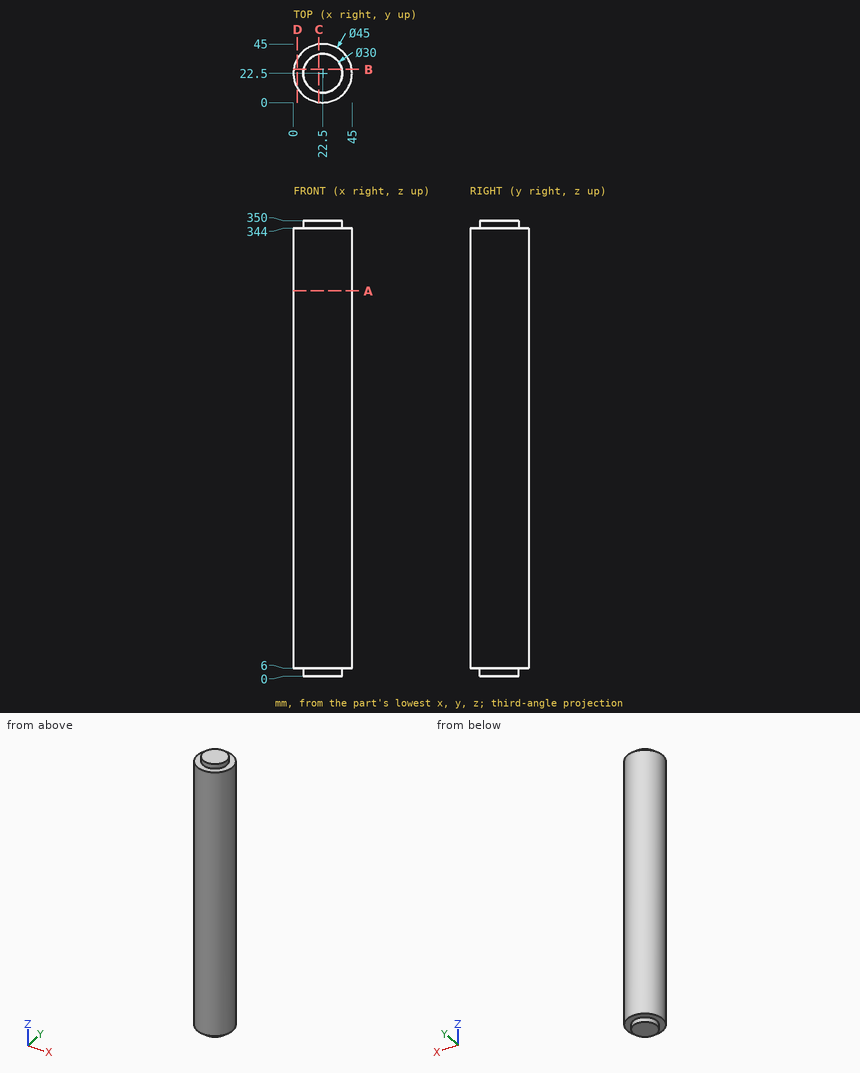
Could you check a few things on this drawing? It's one solid part, dimensions in mm from its lowest x, y, z. Round coordinates to 2 decimals unless told otherwise and drop trailing zeros. Loops run counter-clockwise (first coordinate to the right, second up) from the corner with the lowest first, then second, coordinate; pieces in that order, holes last. Notation, with made-up numbers: M 57,-22 L 84,-22 A19 cw 84,-11 Z; hole C 35.5,69 d4. An arc over 180 degrees is marked long. Write each question's results on one line, items separated by ' | '. Start each with the question number.
(1) If I drill on probe 1 along Y at (x, z) = (22, 235); probe 2 along Z at (x, y) = (3, 18.5), over which ranges is the centre line in solid material (lowest first)? Write a range as from..to.
(2) Will these pins go through, and if not, where does the flat tip stop? P1, Ø3, axis at x = 40, y = 14, coming from the +Z side; P2, Ø3, axis at y = 10.5, z = 256.5, coming from the -X side; P3, Ø1.5, axis at x = 26, z = 54, coming from the -Y side; P4, Ø6, axis at x = 20.5, y = 10, coming from the -Z side.
(3) I want a section at B-B (y = 25.5). Please give me the cut outline in (x, z), then the cut area to 3 significant figures.
(4) I want a section at D-D (x = 3). Please give me the cut outline in (y, z), then the cut area to 3 significant figures.
(5) I want a section at A-A (z = 296). Please give me the cut outline in (x, y), then the cut area to 3 significant figures.
Solved:
1) probe 1: y = 0.01..44.99 | probe 2: z = 6..344
2) P1: stops at z = 344 | P2: stops at x = 2.6 | P3: stops at y = 0.17 | P4: stops at z = 0
3) outline: M 0.2,6 L 7.8,6 L 7.8,0 L 37.2,0 L 37.2,6 L 44.8,6 L 44.8,344 L 37.2,344 L 37.2,350 L 7.8,350 L 7.8,344 L 0.2,344 Z | area: 15,400 mm²
4) outline: M 11.28,6 L 33.72,6 L 33.72,344 L 11.28,344 Z | area: 7,590 mm²
5) outline: C 22.5,22.5 d45 | area: 1,590 mm²
